Autodesk Inventor part; units mm, degrees
ref_plane "YZ Plane" through (0, 0, 0) normal (1, 0, 0) x (0, 1, 0)
ref_plane "XZ Plane" through (0, 0, 0) normal (0, 1, 0) x (-1, 0, 0)
ref_plane "XY Plane" through (0, 0, 0) normal (0, 0, 1) x (1, 0, 0)
sketch "Sketch1" plane through (0, 0, 0) normal (0, 1, 0) x (-1, 0, 0)
  line L0 (32.7591, 186.1581) -> (67.7591, 186.1581)
  arc A0 (72.7591, 181.1581) -> (67.7591, 186.1581) centre (67.7591, 181.1581) ccw
  line L1 (72.7591, 181.1581) -> (72.7591, 171.1581)
  arc A1 (67.7591, 166.1581) -> (72.7591, 171.1581) centre (67.7591, 171.1581) ccw
  line L2 (67.7591, 166.1581) -> (32.7591, 166.1581)
  arc A2 (32.7591, 166.1581) -> (27.7591, 161.1581) centre (32.7591, 161.1581) ccw
  arc A3 (22.7591, 156.1581) -> (27.7591, 161.1581) centre (22.7591, 161.1581) ccw
  line L3 (22.7591, 156.1581) -> (2.7591, 156.1581)
  arc A4 (-2.2409, 161.1581) -> (2.7591, 156.1581) centre (2.7591, 161.1581) ccw
  line L4 (-2.2409, 161.1581) -> (-2.2409, 191.1581)
  arc A5 (2.7591, 196.1581) -> (-2.2409, 191.1581) centre (2.7591, 191.1581) ccw
  line L5 (2.7591, 196.1581) -> (22.7591, 196.1581)
  arc A6 (27.7591, 191.1581) -> (22.7591, 196.1581) centre (22.7591, 191.1581) ccw
  arc A7 (27.7591, 191.1581) -> (32.7591, 186.1581) centre (32.7591, 191.1581) ccw
  circle A8 centre (12.7591, 188.1581) radius 2.6
  circle A9 centre (12.7591, 164.1581) radius 2.6
  circle A10 centre (47.7591, 176.1581) radius 1.6
  point P0 (0, 0)
extrude "Extrusion1" add sketch "Sketch1" along normal blind 6
properties part number "LCD-Plate"
Geometry check sheet. Reference: the model listing, model coordinates, mm. A direction names the side the tool comes from. Coordinates: 2 decimals unless noted, no trailing zeros. Loops run counter-clockwise (first coordinate to the right, second up) from the corner with the lowest first, then second, coordinate; pieces in that order, holes last. Notation, with made-up numbers: (-35, 36.25) - (13, 36.25) arc R16 ccw to (13, 41.25) - close; hole circle Ø2 at (78.5, -12). An arc over 180 degrees is marked (long way). One line per item, written item: value. Start each with the question number.
(1) Cross-section at A-A on z = 189.5. Enter the section's corners in (x, y), plus the area to 3 significant figures.
(2) Cross-section at D-D on x = -44.5. Enter the section's corners in (y, z).
(3) Mould release check, pull along X, two halves, no side actions. Record for faces 4 (the flat face through (-13, 3, 156.158)), 5 (the cylindrical face through (-47.55, 2.96, 174.57)), 6 (the flat face through (2.241, 3, 176)): released by +X, released by -X, zero draft, split by the parting line, or undercut.
(4) Cross-section at C-C on x = -11. Enter the section's corners in (y, z), plus the area to 3 significant figures.
(5) Tool access check on faces 1 (the flat face through (-51, 3, 166.158)), 2 (the cylindrical face through (-12.195, 2.958, 190.696)), 3 (the flat face through (-50, 3, 186.158)). Record the directions out of +Z, -Z, +X, -X, +Y, -Y that give a thin tool (end or side, any length) a straight path to the whole face; none if there is none.
(6) Depth check by flat-ended pin: P1, Ø4.5, axis at x = -12.76, z = 164.16, coming from the -Y side; P2, Ø1.5, axis at y = 3.5, z = 190.5, coming from the -X side; P3, Ø3, axis at x = -57.5, y = 2.5, coming from the -Z side; P4, Ø1.5, axis at y = 1.5, z = 182.5, coming from the -X side. Enter the tip coordinate at first touch or a pass-through.
(7) Material ranges on line 1 (Z direction, x = -13, y = 1.1); line 2 (Z direction, x = -66, y = 4.5); line 3 (X direction, y = 2.4, z = 162), recorded low to high. Write a range as [from, to].
(8) Cross-section at B-B on y = 2.55. Enter the section's corners in (x, z), plus the area to 3 significant figures.
Results below:
1. outline: (-28.04, 0) - (-14.99, 0) - (-14.99, 6) - (-28.04, 6) - close; (-10.53, 0) - (2.24, 0) - (2.24, 6) - (-10.53, 6) - close
1. area: 155 mm2
2. outline: (0, 166.16) - (6, 166.16) - (6, 186.16) - (0, 186.16) - close
3. face 4: zero draft
3. face 5: undercut
3. face 6: released by +X
4. outline: (0, 156.16) - (6, 156.16) - (6, 162.24) - (0, 162.24) - close; (0, 166.07) - (6, 166.07) - (6, 186.24) - (0, 186.24) - close; (0, 190.07) - (6, 190.07) - (6, 196.16) - (0, 196.16) - close
4. area: 194 mm2
5. face 1: -Z, -X, +Y, -Y
5. face 2: +Y, -Y
5. face 3: +Z, -X, +Y, -Y
6. P1: passes through
6. P2: stops at x = -27.96
6. P3: stops at z = 166.16
6. P4: stops at x = -72.72
7. line 1: z = [156.16, 161.57], [166.75, 185.57], [190.75, 196.16]
7. line 2: z = [166.16, 186.16]
7. line 3: x = [-27.83, -14.21], [-11.31, 2.24]
8. outline: (-72.76, 171.16) arc R5 ccw to (-67.76, 166.16) - (-32.76, 166.16) arc R5 cw to (-27.76, 161.16) arc R5 ccw to (-22.76, 156.16) - (-2.76, 156.16) arc R5 ccw to (2.24, 161.16) - (2.24, 191.16) arc R5 ccw to (-2.76, 196.16) - (-22.76, 196.16) arc R5 ccw to (-27.76, 191.16) arc R5 cw to (-32.76, 186.16) - (-67.76, 186.16) arc R5 ccw to (-72.76, 181.16) - close; hole circle Ø3.2 at (-47.76, 176.16); hole circle Ø5.2 at (-12.76, 164.16); hole circle Ø5.2 at (-12.76, 188.16)
8. area: 2,030 mm2
